```python
from build123d import *

# Parameters (mm, degrees)
GEARBOX_START          = -24
PROFILE_1_R            = 18.5
GEARBOX_DEPTH          = 24
THREAD_PILOTS_START    = -3.5
PROFILE_2_R            = 1.25
THREAD_PILOTS_DEPTH    = 3.51
ARMATURE_START         = -53
PROFILE_3_R            = 16.5
ARMATURE_DEPTH         = 29
ENCODER_ENVELOPE_START = -65
PROFILE_4_R            = 15
ENCODER_ENVELOPE_DEPTH = 12
PROFILE_5_R            = 6
NOSE_DEPTH             = 6
OUTPUT_START           = 6
PROFILE_6_R            = 3
OUTPUT_DEPTH           = 15
D_FLAT_START           = 9
PROFILE_7_W            = 8
PROFILE_7_H            = 1.5
D_FLAT_DEPTH           = 12.01


with BuildPart() as part:
    # Profile_1 → Gearbox (new body)
    with BuildSketch(Plane.XY.offset(GEARBOX_START)):
        with Locations((0, -7)):
            Circle(PROFILE_1_R)
    extrude(amount=GEARBOX_DEPTH)

    # Profile_2 → Thread_pilots (cut)
    with BuildSketch(Plane.XY.offset(THREAD_PILOTS_START)):
        with Locations((15.5, -7)):
            Circle(PROFILE_2_R)
        with Locations((7.75, 6.423393759)):
            Circle(PROFILE_2_R)
        with Locations((-7.75, 6.423393759)):
            Circle(PROFILE_2_R)
        with Locations((-15.5, -7)):
            Circle(PROFILE_2_R)
        with Locations((-7.75, -20.423393759)):
            Circle(PROFILE_2_R)
        with Locations((7.75, -20.423393759)):
            Circle(PROFILE_2_R)
    extrude(amount=THREAD_PILOTS_DEPTH, mode=Mode.SUBTRACT)

    # Profile_3 → Armature (add)
    with BuildSketch(Plane.XY.offset(ARMATURE_START)):
        with Locations(Location((0, -7, 0), (0, 0, 180))):
            Circle(PROFILE_3_R)
    extrude(amount=ARMATURE_DEPTH)

    # Profile_4 → Encoder_envelope (add)
    with BuildSketch(Plane.XY.offset(ENCODER_ENVELOPE_START)):
        with Locations((0, -7)):
            Circle(PROFILE_4_R)
    extrude(amount=ENCODER_ENVELOPE_DEPTH)

    # Profile_5 → Nose (add)
    with BuildSketch(Plane.XY):
        Circle(PROFILE_5_R)
    extrude(amount=NOSE_DEPTH)

    # Profile_6 → Output (add)
    with BuildSketch(Plane.XY.offset(OUTPUT_START)):
        Circle(PROFILE_6_R)
    extrude(amount=OUTPUT_DEPTH)

    # Profile_7 → D_flat (cut)
    with BuildSketch(Plane.XY.offset(D_FLAT_START)):
        with Locations((0, 3.25)):
            Rectangle(PROFILE_7_W, PROFILE_7_H)
    extrude(amount=D_FLAT_DEPTH, mode=Mode.SUBTRACT)


solid = part.part
```
Work out the finished part from the listing and answer in its coordinate system (mm). A direction names the side the tool comes from. Round coordinates to 2 decimals unless told otherwise and drop trailing zeros. Loops run counter-clockwise (first coordinate to the right, second up) from the corner with the lowest first, then second, coordinate; pieces in that order, holes last.
(1) The part is cut by section D-D, the plane y = -13.5. Give the vertices of the cut face in (x, z), and give its area (3 significant figures).
Computed values:
outline: (-17.32, -24) - (-15.17, -24) - (-15.17, -53) - (-13.52, -53) - (-13.52, -65) - (13.52, -65) - (13.52, -53) - (15.17, -53) - (15.17, -24) - (17.32, -24) - (17.32, 0) - (-17.32, 0) - close
area: 2,040 mm2
(2) For faces 4 (the flat face through (0, -7, -65)), 5 (the flat face through (-4, 8, -53)), 6 (the cylindrical face through (-14.68, -18.26, -12.17)), 7 (the cylindrical face through (-8.67, -19.58, -1.77)), 8 (the flat face through (0, 2.5, 15)), determine the directions among +Z, -Z, +X, -X, +Y, -Y from which every point of the face is accessible in a straight line to the end or side of a thin tool.
Computed values:
face 4: -Z, +X, -X, +Y, -Y
face 5: -Z
face 6: +Z, -Z
face 7: +Z
face 8: +Z, +X, -X, +Y
(3) Find the intervals of material crossed by L1, parallel to Z at x = -13, y = -11.5; L2, parallel to Y at x = -15, z = -2; L3, parallel to Y at x = 15.5, z = -1.1, in increasing order.
Computed values:
L1: z = -65 to 0
L2: y = -17.83 to -8.15, -5.85 to 3.83
L3: y = -17.1 to -8.25, -5.75 to 3.1
(4) The part is cut by section B-B, the plane x = -7.75. Give the vertices of the cut face in (y, z), and give its area (3 significant figures).
Computed values:
outline: (-23.8, -24) - (-21.57, -24) - (-21.57, -53) - (-19.84, -53) - (-19.84, -65) - (5.84, -65) - (5.84, -53) - (7.57, -53) - (7.57, -24) - (9.8, -24) - (9.8, 0) - (7.67, 0) - (7.67, -3.5) - (5.17, -3.5) - (5.17, 0) - (-19.17, 0) - (-19.17, -3.5) - (-21.67, -3.5) - (-21.67, 0) - (-23.8, 0) - close
area: 1,940 mm2
(5) The part is cut by section A-A, the plane y = -7. Give the vertices of the cut face in (x, z), and give its area (3 significant figures).
Computed values:
outline: (-18.5, -24) - (-16.5, -24) - (-16.5, -53) - (-15, -53) - (-15, -65) - (15, -65) - (15, -53) - (16.5, -53) - (16.5, -24) - (18.5, -24) - (18.5, 0) - (16.75, 0) - (16.75, -3.5) - (14.25, -3.5) - (14.25, 0) - (-14.25, 0) - (-14.25, -3.5) - (-16.75, -3.5) - (-16.75, 0) - (-18.5, 0) - close
area: 2,190 mm2
(6) The mould has two halves that part along X. Classify faces 1 (the cylindrical face through (-6, 0, 3)), 2 (the flat face through (0, -7, 0)), 3 (the flat face through (-8, 6, -3.5)): pulls with the +X half, pulls with the -X half, needs draft (parallel to the pull), parting line crosses it, or undercut.
Computed values:
face 1: parting line crosses it
face 2: needs draft
face 3: undercut
(7) The part is cut by section C-C, the plane z = -19. Give the vertices of the cut face in (x, y).
Computed values:
outline: circle Ø37 at (0, -7)
(8) Each of these flat-tipped pins is pushed along its axis until it touches: P1, Ø2.5, axis at x = 0.5, z = 15, coming from the +Y side; P2, Ø3, axis at x = 15.5, y = -7.5, coming from the +Z side; P3, Ø6, axis at x = -6.5, z = -48, coming from the +Y side; P4, Ø18.5, axis at x = 4.5, y = 0.5, coming from the +Z side. Where does it stop, or does it pass through?
Computed values:
P1: stops at y = 2.5
P2: stops at z = 0
P3: stops at y = 9.12
P4: stops at z = 21
